The model under review builds one solid part; all positions refer to its coordinate system, in mm. A direction names the side the tool comes from. Coordinates: 2 decimals unless noted, no trailing zeros. Order: outer loops, then holes, each group sorted by start corner. A loop starts at its lowest first (then second) coordinate and runs counter-clockwise, first axis right, second up. Notation, with made-up numbers: M 5,73.25 L 45,73.25 A20 ccw 45,92.25 Z; hole C 41.25,-33 d11. An arc over 180 degrees is marked long. Answer in a Markdown table with one row per item.
from build123d import *

# Parameters (mm, degrees)
F0_W     = 9
F0_H     = 4
F0_H_2   = 6.5
F1_DEPTH = 10
F2_R     = 0.5
F3_R     = 1
F4_DEPTH = 25


with BuildPart() as f1:
    # F0 (on Front) → F1 (new body)
    with BuildSketch(Plane.XZ):
        with BuildLine():
            ThreePointArc((-7.5, -3.6921049214), (-3.753158649, -3.9229938263), (0, -4))
            Line((0, -4), (0, -2.5))
            Line((0, -2.5), (-7.5, -2.5))
            Line((-7.5, -2.5), (-7.5, -3.6921049214))
        make_face()
        with BuildLine():
            Line((0, -2.5), (0, -4))
            ThreePointArc((0, -4), (3.753158649, -3.9229938263), (7.5, -3.6921049214))
            Line((7.5, -3.6921049214), (7.5, -2.5))
            Line((7.5, -2.5), (0, -2.5))
        make_face()
        with BuildLine():
            Line((7.5, -2.5), (7.5, -3.6921049214))
            ThreePointArc((7.5, -3.6921049214), (12.0147941529, -3.2077434482), (16.5, -2.5))
            Line((16.5, -2.5), (7.5, -2.5))
        make_face()
        Polygon((-7.5, -2.5), (0, -2.5), (7.5, -2.5), (7.5, 4), (-7.5, 4), align=None)
        Rectangle(F0_W, F0_H, mode=Mode.SUBTRACT)
        with BuildLine():
            ThreePointArc((-16.5, -2.5), (-12.0147941529, -3.2077434482), (-7.5, -3.6921049214))
            Line((-7.5, -3.6921049214), (-7.5, -2.5))
            Line((-7.5, -2.5), (-16.5, -2.5))
        make_face()
        with Locations((12, 0.75)):
            Rectangle(F0_W, F0_H_2)
        with Locations((-12, 0.75)):
            Rectangle(F0_W, F0_H_2)
    extrude(amount=F1_DEPTH)

    # F2 (call 1 of 5: OpenCascade refuses the feature's edges together)
    f2_edges = [f1.edges().sort_by_distance(p)[0] for p in [
        (16.5, -5, 4),
        (-16.5, -5, 4),
        (0, -10, 4),
        (0, 0, 4),
    ]]
    fillet(f2_edges, radius=F2_R)

    # F2#2 (call 2 of 5)
    f2_2_edges = [f1.edges().sort_by_distance(p)[0] for p in [
        (16.5, -5, -2.5),
    ]]
    fillet(f2_2_edges, radius=F2_R)

    # F2#3 (call 3 of 5)
    f2_3_edges = [f1.edges().sort_by_distance(p)[0] for p in [
        (-16.5, -5, -2.5),
    ]]
    fillet(f2_3_edges, radius=F2_R)

    # F2#4 (call 4 of 5)
    f2_4_edges = [f1.edges().sort_by_distance(p)[0] for p in [
        (-4.5, 0, 0),
        (0, 0, 2),
        (4.5, 0, 0),
        (0, 0, -2),
    ]]
    fillet(f2_4_edges, radius=F2_R)

    # F2#5 (call 5 of 5)
    f2_5_edges = [f1.edges().sort_by_distance(p)[0] for p in [
        (-4.5, -10, 0),
        (0, -10, 2),
        (4.5, -10, 0),
        (0, -10, -2),
    ]]
    fillet(f2_5_edges, radius=F2_R)

    # F3 (on face) → F4 (cut)
    with BuildSketch(Plane.XY.offset(4)):
        with Locations((-12, -5)):
            Circle(F3_R)
        with Locations((12, -5)):
            Circle(F3_R)
    extrude(amount=-F4_DEPTH, mode=Mode.SUBTRACT)


solid = f1.part
(1) Take a section at A-A (z = 0.75). Write out the cut boundary in (x, y).
Report:
| item | result |
|---|---|
| outline | M -16.5,-10 L -5,-10 A0.5 ccw -4.5,-9.5 L -4.5,-0.5 A0.5 ccw -5,0 L -16.5,0 Z; M 4.5,-9.5 A0.5 ccw 5,-10 L 16.5,-10 L 16.5,0 L 5,0 A0.5 ccw 4.5,-0.5 Z; hole C -12,-5 d2; hole C 12,-5 d2 |
(2) Insertion check: P1, Ø2.5, axis at x = 12, y = -5, coming from the -Z side; P2, Ø4, axis at x = -10, y = -2.5, coming from the -Z side. Each pin has a flat end and moves straight along its axis. Give the tip position at first contact, or say it passes through.
Report:
| item | result |
|---|---|
| P1 | z = -3.37 |
| P2 | z = -3.65 |
(3) Machinability: for faces 1 (the flat face through (0, 0, -3)), 2 (the flat face through (0, -5, -2)), which of the approach directions +Z, -Z, +X, -X, +Y, -Y give a long, thin tool a straight path to every point of the face, cutting with its end or side? Answer none if there is none.
Report:
| item | result |
|---|---|
| face 1 | +Z, -Z, +X, -X, +Y |
| face 2 | +Y, -Y |
(4) The part is to be moulded in two halves that separate along Z. For faces 3 (the flat face through (16.5, -5, 1)), 4 (the flat face through (0, -5, 4)), 5 (the flat face through (0, -5, 2)), say which applies: +Z half, -Z half, draft (parallel to the pull), parting line (faces both ways), or undercut.
Report:
| item | result |
|---|---|
| face 3 | draft |
| face 4 | +Z half |
| face 5 | undercut |
(5) Take a section at D-D (x = -12). Write out the cut boundary in (y, z), then the cut area to 3 significant figures.
Report:
| item | result |
|---|---|
| outline | M -10,-3.21 L -6,-3.21 L -6,4 L -9.5,4 A0.5 ccw -10,3.5 Z; M -4,-3.21 L 0,-3.21 L 0,3.5 A0.5 ccw -0.5,4 L -4,4 Z |
| area | 57.6 mm^2 |
(6) To check wall thickness, follow line 1 (X direction, y = -5, z = 2.25); line 2 (X direction, y = -5, z = -1); line 3 (Z direction, x = 1, y = -3.5). State the ranges of each line that lie inside material, in increasing order. Write a range as [from, to].
Report:
| item | result |
|---|---|
| line 1 | [-16.5, -13], [-11, 11], [13, 16.5] |
| line 2 | [-16.5, -13], [-11, -4.5], [4.5, 11], [13, 16.5] |
| line 3 | [-3.99, -2], [2, 4] |
(7) Take a section at C-C (y = -5). Write out the cut boundary in (x, z), then the cut area to 3 significant figures.
Report:
| item | result |
|---|---|
| outline | M -16.5,-2.08 A0.5 ccw -16.09,-2.57 A91.5 ccw -13,-3.07 L -13,4 L -16,4 A0.5 ccw -16.5,3.5 Z; M -11,-3.34 A91.5 ccw 11,-3.34 L 11,4 L -11,4 Z; M 13,-3.07 A91.5 ccw 16.09,-2.57 A0.5 ccw 16.5,-2.08 L 16.5,3.5 A0.5 ccw 16,4 L 13,4 Z; hole M -4.5,-2 L 4.5,-2 L 4.5,2 L -4.5,2 Z |
| area | 183 mm^2 |
(8) Take a section at B-B (y = -7.5). Write out the cut boundary in (x, z).
Report:
| item | result |
|---|---|
| outline | M -16.5,-2.08 A0.5 ccw -16.09,-2.57 A91.5 ccw 16.09,-2.57 A0.5 ccw 16.5,-2.08 L 16.5,3.5 A0.5 ccw 16,4 L -16,4 A0.5 ccw -16.5,3.5 Z; hole M -4.5,-2 L 4.5,-2 L 4.5,2 L -4.5,2 Z |
